Verification items for the finished model (mm, model axes). A direction names the side the tool comes from. Coordinates: 2 decimals unless noted, no trailing zeros. Write each loop counter-clockwise with the first axis right and the second up, starting at its lowest first coordinate (ties: lowest second). Pieces come first, ordered by that corner, then holes. Notation, with made-up numbers: (51, 72) -> (70, 72) arc R20 cw to (70, 80) -> close; hole circle Ø10 at (-26.5, -28). An arc over 180 degrees is marked (long way). Answer in a Markdown table with one row per item.
```python
from build123d import *

# Parameters (mm, degrees)
F0_R      = 5
F1_DEPTH  = 100
F2_W      = 50
F2_H      = 50
F3_DEPTH  = 10
F4_R      = 2.5
F5_DEPTH  = 2.5
F6_R      = 10
F7_DEPTH  = 5
F8_R      = 10
F9_DEPTH  = 5
F10_R     = 2.5
F11_DEPTH = 2.5
F12_R     = 10
F13_DEPTH = 5
F14_R     = 10
F15_DEPTH = 5
F20_DEPTH = 2.5
F24_DEPTH = 2.5
F26_DEPTH = 2.5


with BuildPart() as f1:
    # F0 (on Top) → F1 (new body)
    with BuildSketch(Plane.XY):
        Circle(F0_R)
    extrude(amount=F1_DEPTH)

    # F2 (on Top) → F3 (join)
    with BuildSketch(Plane.XY):
        Rectangle(F2_W, F2_H)
    extrude(amount=-F3_DEPTH)

    # F4 (on face) → F5 (join)
    with BuildSketch(Plane.YZ.offset(25)):
        with Locations((-20, -5)):
            Circle(F4_R)
        with Locations((20, -5)):
            Circle(F4_R)
    extrude(amount=F5_DEPTH)

    # F6 (on face) → F7 (join)
    with BuildSketch(Plane.YZ.offset(27.5)):
        with Locations((-20, -5)):
            Circle(F6_R)
    extrude(amount=F7_DEPTH)

    # F8 (on face) → F9 (join)
    with BuildSketch(Plane.YZ.offset(27.5)):
        with Locations((20, -5)):
            Circle(F8_R)
    extrude(amount=F9_DEPTH)

    # F10 (on face) → F11 (join)
    with BuildSketch(Plane(origin=(-25, 0, 0), x_dir=(0, -1, 0), z_dir=(-1, 0, 0))):
        with Locations((-20, -5)):
            Circle(F10_R)
        with Locations((20, -5)):
            Circle(F10_R)
    extrude(amount=F11_DEPTH)

    # F12 (on face) → F13 (join)
    with BuildSketch(Plane(origin=(-27.5, 0, 0), x_dir=(0, -1, 0), z_dir=(-1, 0, 0))):
        with Locations((-20, -5)):
            Circle(F12_R)
    extrude(amount=F13_DEPTH)

    # F14 (on face) → F15 (join)
    with BuildSketch(Plane(origin=(-27.5, 0, 0), x_dir=(0, -1, 0), z_dir=(-1, 0, 0))):
        with Locations((20, -5)):
            Circle(F14_R)
    extrude(amount=F15_DEPTH)

    # F19 (on 3pt) → F20 (join, symmetric)
    with BuildSketch(Plane(origin=(0, 0, 0), x_dir=(0.7071067812, 0.7071067812, 0), z_dir=(0.7071067812, -0.7071067812, 0))):
        Polygon((-5.5, 20), (-35.3553390593, 0), (-5.5, 0), align=None)
    extrude(amount=F20_DEPTH, both=True)

    # F23 (on 3pt) → F24 (join, symmetric)
    with BuildSketch(Plane(origin=(0, 0, 0), x_dir=(-0.7071067812, 0.7071067812, 0), z_dir=(0.7071067812, 0.7071067812, 0))):
        Polygon((5.5, 20), (5.5, 0), (35.3553390593, 0), align=None)
        Polygon((-35.3553390593, 0), (-5.5, 0), (-5.5, 20), align=None)
    extrude(amount=F24_DEPTH, both=True)

    # F25 (on 3pt) → F26 (join, symmetric)
    with BuildSketch(Plane(origin=(0, 0, 0), x_dir=(0.7071067812, 0.7071067812, 0), z_dir=(0.7071067812, -0.7071067812, 0))):
        Polygon((5.5, 20), (5.5, 0), (35.3553390593, 0), align=None)
    extrude(amount=F26_DEPTH, both=True)


solid = f1.part
```
1. Thickness scan on line 1 (X direction, y = 17, z = -3); line 2 (Z direction, x = 24.5, y = -17.5); line 3 (X direction, y = -1, z = -5). Record the ranges inside material, lowest first. Write a range as from..to.
Geometry says:
| item | result |
|---|---|
| line 1 | -32.5..-27.5, -25..25, 27.5..32.5 |
| line 2 | -10..0 |
| line 3 | -25..25 |
2. Section check D-D, the plane z = 57. Record the boundary of the cut face in (x, y).
Geometry says:
| item | result |
|---|---|
| outline | circle Ø10 at (0, 0) |
3. Mould release check, pull along X, two halves, no side actions. Record for faces 5 (the cylindrical face through (-29.96, -29.54, -2)), 6 (the flat face through (3.914, 3.864, 10.14)), 7 (the flat face through (3.914, -3.864, 9.86)), 8 (the flat face through (-32.5, -20, -5)): released by +X, released by -X, zero draft, split by the parting line, or undercut.
Geometry says:
| item | result |
|---|---|
| face 5 | zero draft |
| face 6 | undercut |
| face 7 | undercut |
| face 8 | released by -X |
4. Section check A-A, the plane y = 0. Record the boundary of the cut face in (x, z), plus the area to 3 significant figures.
Geometry says:
| item | result |
|---|---|
| outline | (-25, -10) -> (25, -10) -> (25, 0) -> (5, 0) -> (5, 100) -> (-5, 100) -> (-5, 0) -> (-25, 0) -> close |
| area | 1,500 mm^2 |
5. Section check C-C, the plane y = -15. Record the boundary of the cut face in (x, z).
Geometry says:
| item | result |
|---|---|
| outline | (-32.5, -13.66) -> (-27.5, -13.66) -> (-27.5, 3.66) -> (-32.5, 3.66) -> close; (-25, -10) -> (25, -10) -> (25, 0) -> (18.54, 0) -> (18.54, 7.8) -> (11.46, 11.15) -> (11.46, 0) -> (-11.46, 0) -> (-11.46, 11.15) -> (-18.54, 7.8) -> (-18.54, 0) -> (-25, 0) -> close; (27.5, -13.66) -> (32.5, -13.66) -> (32.5, 3.66) -> (27.5, 3.66) -> close |
6. Tool access check on faces 1 (the flat face through (0, 6, 0)), 2 (the flat face through (0, 25, -5)), 3 (the flat face through (14.617, 14.568, 9.86)), 4 (the flat face through (-27.5, -22, -7)). Record the directions out of +Z, -Z, +X, -X, +Y, -Y that give a thin tool (end or side, any length) a straight path to the whole face; none if there is none.
Geometry says:
| item | result |
|---|---|
| face 1 | +Z |
| face 2 | -Z, +Y |
| face 3 | +Z, +Y |
| face 4 | none |
7. Depth check by flat-ended pin: P1, Ø0.9, axis at x = -26, y = -23.5, coming from the -Z side; P2, Ø1.4, axis at x = 25.5, y = 22.5, coming from the -Z side; P3, Ø8, axis at x = 12, z = -7.5, coming from the -Y side; P4, Ø1.5, axis at x = -6.5, z = 59, coming from the +Y side. Enter the tip coordinate at first touch or a pass-through.
Geometry says:
| item | result |
|---|---|
| P1 | z = 0 |
| P2 | z = -10 |
| P3 | y = -25 |
| P4 | through |
